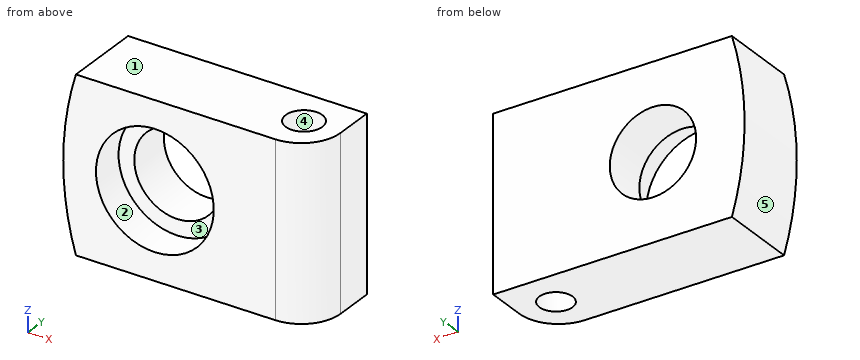
```python
from build123d import *

# Parameters (mm, degrees)
BOSS_EXTRUDE1_DEPTH = 30
SKETCH2_R           = 22.5
CUT_EXTRUDE1_DEPTH  = 13
SKETCH3_R           = 16.5
CUT_EXTRUDE2_DEPTH  = 61.679485825
FILLET1_R           = 15


with BuildPart() as part:
    # Sketch1 → Boss-Extrude1 (new body)
    with BuildSketch(Plane(origin=(0, 0, 0), x_dir=(1, 0, 0), z_dir=(0, 1, 0))):
        with BuildLine():
            ThreePointArc((-43.163514831, 33), (-48, 0), (-43.163514831, -33))
            Line((-43.163514831, -33), (48, -33))
            Line((48, -33), (48, 33))
            Line((48, 33), (-43.163514831, 33))
        make_face()
    extrude(amount=BOSS_EXTRUDE1_DEPTH)

    # Sketch2 → Cut-Extrude1 (cut)
    with BuildSketch(Plane.XZ):
        with Locations(Location((-13, 0, 0), (0, 0, 270))):
            Circle(SKETCH2_R)
    extrude(amount=-CUT_EXTRUDE1_DEPTH, mode=Mode.SUBTRACT)

    # Sketch3 → Cut-Extrude2 (cut, through all)
    with BuildSketch(Plane.XZ.offset(-13)):
        with Locations(Location((-13, 0, 0), (0, 0, 270))):
            Circle(SKETCH3_R)
    extrude(amount=-CUT_EXTRUDE2_DEPTH, mode=Mode.SUBTRACT)

    # Fillet1
    fillet1_edges = [part.edges().sort_by_distance(p)[0] for p in [
        (48, 0, 0),
    ]]
    fillet(fillet1_edges, radius=FILLET1_R)

    # Sketch4 → Cut-Revolve1 (revolve, cut)
    with BuildSketch(Plane(origin=(0, 15, 0), x_dir=(1, 0, 0), z_dir=(0, 1, 0)), mode=Mode.PRIVATE) as cut_revolve1_sk:
        Polygon((41, -33), (40.34, 33), (34, 33), (34, -33), align=None)
    revolve(cut_revolve1_sk.sketch.rotate(Axis((34, 15, -33), (0, 0, 1)), 180), axis=Axis((34, 15, -33), (0, 0, 1)), mode=Mode.SUBTRACT)


solid = part.part
```
Design review of the part built by this model. Coordinates are the model's own, in mm. Face numbers are marked on the shaded views. A direction names the side the tool comes from. Give positions to 0.01 mm unless a question says otherwise; leave off trailing zeros. Loops run counter-clockwise (first coordinate to the right, second up) from the corner with the lowest first, then second, coordinate; pieces in that order, holes last. Notation, with made-up numbers: M 22.5,67.5 L 45.5,67.5 A19 ccw 45.5,81.5 Z; hole C -20,8.25 d10. An arc over 180 degrees is marked long. Return JSON: item names as keys, results as strings. Group by question number.
Item 1: We need section C-C (y = 25). Give the boundary of the cut face in (x, z).
Item 2: For probe 1 along X at (y, z) = (23.5, 0); probe 2 along Y at (x, z) = (7.5, -5); probe 3 along X at (y, z) = (8, -9), list the stretches that pass through material, from the lowest coordinate up.
Item 3: We need section D-D (z = 19.5). Give the boundary of the cut face in (x, y) (3 decimals).
Item 4: We need section A-A (x = -13). Give the boundary of the cut face in (y, z).
Item 5: Tool access review of the marked faces 1 and 2: name each direction out of +Z, -Z, +X, -X, +Y, -Y from which nothing blocks a thin tool from reaching the whole face with its end or side.
Item 6: Mouldability with a two-part tool opening along Y and no side actions: class the marked faces 3, 4 and 5 as released by +Y, released by -Y, zero draft, split by the parting line, or undercut.
Item 7: We need section B-B (z = 0). Give the boundary of the cut face in (x, y), and give its area (3 significant figures).
Item 8: Insertion check: pin 1 Ø5 at (y, z) = (7, 13) entering from -X; pin 2 Ø3 at (x, z) = (-17.5, -19) entering from -Y; pin 3 Ø6 at (y, z) = (3.5, -9) entering from -X; pin 4 Ø3 at (y, z) = (14, 9) entering from +X. Each pin has a flat end and moves straight along its axis. Give the tip position at first contact, or say it passes through.
Output:
{
 "1": {"outline": "M -43.16,-33 L 48,-33 L 48,33 L -43.16,33 A115 ccw Z; hole C -13,0 d33"},
 "2": {"probe 1": "x = -48 to -29.5, 3.5 to 48", "probe 2": "y = 13 to 30", "probe 3": "x = -47.65 to -33.62, 7.62 to 46.27"},
 "3": {"outline": "M -46.335,0 L -24.225,0 L -24.225,13 L -1.775,13 L -1.775,0 L 33,0 A15 ccw 48,15 L 48,30 L -46.335,30 Z; hole C 34,15 d13.73"},
 "4": {"outline": "M 0,-33 L 30,-33 L 30,-16.5 L 13,-16.5 L 13,-22.5 L 0,-22.5 Z; M 0,22.5 L 13,22.5 L 13,16.5 L 30,16.5 L 30,33 L 0,33 Z"},
 "5": {"face 1": "+Z, +X, -X, +Y, -Y", "face 2": "-Y"},
 "6": {"face 3": "released by -Y", "face 4": "undercut", "face 5": "zero draft"},
 "7": {"outline": "M -48,0 L -35.5,0 L -35.5,13 L -29.5,13 L -29.5,30 L -48,30 Z; M 3.5,13 L 9.5,13 L 9.5,0 L 33,0 A15 ccw 48,15 L 48,30 L 3.5,30 Z; hole C 34,15 d13.34", "area": "1,550 mm^2"},
 "8": {"pin 1": "stops at x = -47.52", "pin 2": "stops at y = 13", "pin 3": "stops at x = -47.84", "pin 4": "stops at x = 48"}
}
